from build123d import *

# Parameters (mm, degrees)
SKETCH_R     = 1.7
PAD_DEPTH    = 1.4
SKETCH001_R  = 7.5
PAD001_DEPTH = 11
SKETCH002_R  = 7
POCKET_DEPTH = 7
FILLET_R     = 0.5
SKETCH004_W  = 0.8
SKETCH004_H  = 4.972782
PAD002_DEPTH = 8


with BuildPart() as part:
    # Sketch → Pad (new body)
    with BuildSketch(Plane.XZ):
        with BuildLine():
            Line((5.369565, 7.836949), (13.195652, 2.474826))
            ThreePointArc((13.195652, -2.474826), (14.5, 0), (13.195652, 2.474826))
            Line((13.195652, -2.474826), (5.369565, -7.836949))
            ThreePointArc((-5.369565, -7.836949), (0, -9.5), (5.369565, -7.836949))
            Line((-5.369565, -7.836949), (-13.195652, -2.474826))
            ThreePointArc((-13.195652, 2.474826), (-14.5, 0), (-13.195652, -2.474826))
            Line((-13.195652, 2.474826), (-5.369565, 7.836949))
            ThreePointArc((5.369565, 7.836949), (0, 9.5), (-5.369565, 7.836949))
        make_face()
        with Locations((11.5, 0)):
            Circle(SKETCH_R, mode=Mode.SUBTRACT)
        with Locations((-11.5, 0)):
            Circle(SKETCH_R, mode=Mode.SUBTRACT)
    extrude(amount=PAD_DEPTH)

    # Sketch001 → Pad001 (join)
    with BuildSketch(Plane.XZ):
        Circle(SKETCH001_R)
    extrude(amount=-PAD001_DEPTH)

    # Sketch002 (on Face5 of Pad001) → Pocket (cut)
    with BuildSketch(Plane.XZ.offset(1.4)):
        Circle(SKETCH002_R)
        with BuildLine():
            ThreePointArc((-1.5, 5.550901), (0, -5.75), (1.5, 5.550901))
            Line((1.5, 5.550901), (1.5, 2.75))
            Line((1.5, 2.75), (-1.5, 2.75))
            Line((-1.5, 2.75), (-1.5, 5.550901))
        make_face(mode=Mode.SUBTRACT)
    extrude(amount=-POCKET_DEPTH, mode=Mode.SUBTRACT)

    # Fillet
    fillet_edges = [part.edges().sort_by_distance(p)[0] for p in [
        (0, -1.4, 9.5),
        (-9.282609, -1.4, 5.155887),
        (-14.5, -1.4, 0),
        (-9.282609, -1.4, -5.155887),
        (0, -1.4, -9.5),
        (9.282609, -1.4, -5.155887),
        (14.5, -1.4, 0),
        (9.282609, -1.4, 5.155887),
        (-7.5, 11, 0),
        (-7, -1.4, 0),
    ]]
    fillet(fillet_edges, radius=FILLET_R)

    # Sketch004 (on Face25 of Fillet) → Pad002 (join)
    with BuildSketch(Plane(origin=(0, 11, 0), x_dir=(1, 0, 0), z_dir=(0, 1, 0))):
        Polygon((2.999739, 0.039573), (7.918946, 0.767563), (7.80183, 1.558944), (2.882623, 0.830954), align=None)
        Polygon((2.512335, -1.639565), (1.989694, -2.245244), (5.754578, -5.493969), (6.277219, -4.88829), align=None)
        with Locations((0, -5.459605)):
            Rectangle(SKETCH004_W, SKETCH004_H)
        Polygon((-5.754578, -5.493969), (-6.277219, -4.88829), (-2.512335, -1.639565), (-1.989694, -2.245244), align=None)
        Polygon((-2.999739, 0.039573), (-7.918946, 0.767563), (-7.80183, 1.558944), (-2.882623, 0.830954), align=None)
    extrude(amount=PAD002_DEPTH)


solid = part.part
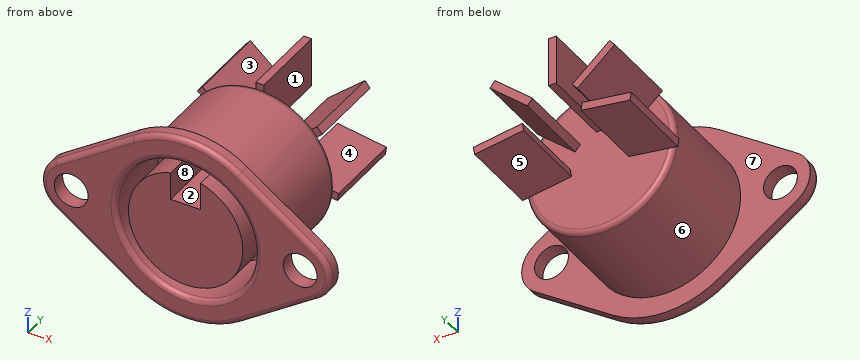
Read the model definition and answer for the solid it produces. Units are mm, in the model's axes. Face numbers are marked on the shaded views. A direction names the side the tool comes from. Round coordinates to 2 decimals unless told otherwise and drop trailing zeros. Loops run counter-clockwise (first coordinate to the right, second up) from the corner with the lowest first, then second, coordinate; pieces in that order, holes last. Notation, with made-up numbers: (-28, 57) - (15, 57) arc R17 cw to (15, 70) - close; hole circle Ø7 at (46.25, -25.75). An arc over 180 degrees is marked (long way). One line per question, with ' | ' between items. Start each with the question number.
Q1. Find the intervals of material crossed by L1, parallel to Z at x = 0, y = 0.75; L2, parallel to X at y = -0.25, z = 4.5; L3, parallel to X at y = 1.75, z = 2.25, in increasing order.
Q2. Section B-B on z = 1.25 is taken. Count the separate pieces of the cut face and the enclosed holes in it, plus the area to 3 significant figures.
Q3. For a pull along Z with two mould halves and no side action, classify the marked faces 6, 7 and 8 as +Z half, -Z half, draft (parallel to the pull), parting line (faces both ways), or undercut.
Q4. Section A-A on x = 0 is taken. Give the vertices of the cut face in (y, z).
Q5. For the marked faces 1, 2, 3, 4 and 5, determine the directions among +Z, -Z, +X, -X, +Y, -Y from which every point of the face is accessible in a straight line to the end or side of a thin tool.
Q6. Flat-ended cylindrical pins translate along their axes: pin 1 (0.9 mm diameter, centred on x = 0.5, y = 3.5, fed in from +Z); pin 2 (8 mm diameter, centred on y = 16, z = -2.5, fed in from -X); pin 3 (5.5 mm diameter, centred on y = 13.5, z = 4.5, fed in from +X). Find the tip coordinate at first contact, or state that the pin passes through.
Established:
1) L1: -7.5 to -7, -5.75 to 2.75, 7 to 7.5 | L2: -10.24 to -5.36, -3.58 to -1.5, 1.5 to 3.58, 5.36 to 10.24 | L3: -7.15 to -6.63, -5.29 to 5.29, 6.63 to 7.15
2) separate pieces: 3 | enclosed holes: 0 | area: 178 mm²
3) face 6: parting line | face 7: draft | face 8: undercut
4) outline: (-1.4, -9) arc R0.5 ccw to (-0.9, -9.5) - (0, -9.5) - (0, -7.5) - (10.5, -7.5) arc R0.5 ccw to (11, -7) - (11, 2.97) - (19, 2.97) - (19, 7.95) - (11, 7.95) - (11, 7) arc R0.5 ccw to (10.5, 7.5) - (0, 7.5) - (0, 9.5) - (-0.9, 9.5) arc R0.5 ccw to (-1.4, 9) - (-1.4, 7.5) arc R0.5 ccw to (-0.9, 7) - (5.6, 7) - (5.6, 2.75) - (-1.4, 2.75) - (-1.4, -5.75) - (5.6, -5.75) - (5.6, -7) - (-0.9, -7) arc R0.5 ccw to (-1.4, -7.5) - close
5) face 1: +Z, -Z, +Y | face 2: -Y | face 3: +Z, +Y | face 4: +X, +Y | face 5: -Z, +Y
6) pin 1: z = 7.5 | pin 2: x = -7.92 | pin 3: x = 6.35
